The listing builds one solid part. Answer for the finished solid, in the listing's coordinates (mm). A direction names the side the tool comes from. Round coordinates to 2 decimals unless told otherwise and drop trailing zeros. Write each loop counter-clockwise with the first axis right and the second up, starting at its lowest first coordinate (ties: lowest second). Pieces come first, ordered by that corner, then holes.
Item 1: This flat-tipped pin is pushed along its axis until it touches: pin 1 (3 mm diameter, centred on x = 44.5, z = 173.5, fed in from -Y). Where does it stop, or does it pass through?
Item 2: For a pull along X with two mould halves and no side action, classify faces 1 (the face through (68, 0, 132)), 2 (the face through (59, 3, 267)) as +X half, -X half, draft (parallel to the pull), parting line (faces both ways), or undercut.
Item 3: A tool of negligible diameter and unlimited length cuts with its end or side. For faces 3 (the face through (59, 3, 0)), 4 (the face through (95.24, -13, 135)), from which of +Z, -Z, +X, -X, +Y, -Y can it reach the whole face along a straight path? Write none if from no direction.
Item 4: Find the intervals of material crossed by probe 1 along Y at (x, z) = (39, 163), in increasing order.
Item 5: Find section A-A on y = -11.5. Give the number of separate pieces and of enclosed holes in the cut face, then the cut area to 3 significant figures.
Item 6: Find section B-B on x = 53. Give the vertices of the cut face in (y, z).
Autodesk Inventor part; units mm, degrees
ref_plane "YZ Plane" through (0, 0, 0) normal (1, 0, 0) x (0, 1, 0)
ref_plane "XZ Plane" through (0, 0, 0) normal (0, 1, 0) x (-1, 0, 0)
ref_plane "XY Plane" through (0, 0, 0) normal (0, 0, 1) x (1, 0, 0)
sketch "Sketch4" plane through (0, 0, 0) normal (0, 0, 1) x (1, 0, 0)
  line L0 (0, 0) -> (97.04, 0)
  line L1 (97.04, 0) -> (97.04, 7.8)
  line L2 (97.04, 7.8) -> (0, 7.8)
  line L3 (0, 7.8) -> (0, 0)
  dimension "d15" = 97.04
  dimension "d16" = 7.8
extrude "Extrusion3" add sketch "Sketch4" along normal blind 267
sketch "Sketch5" plane through (0, 0, 267) normal (0, 0, 1) x (1, 0, 0)
  line L0 (0, 0) -> (97.04, 0)
  line L1 (0, 0) -> (1.8, 0)
  line L2 (1.8, 0) -> (1.8, -25.2)
  line L3 (1.8, -25.2) -> (0, -25.2)
  line L4 (0, -25.2) -> (0, 0)
  line L5 (9.7367, 0) -> (9.7367, -25.2)
  line L6 (7.9367, 0) -> (9.7367, 0)
  line L7 (7.9367, -25.2) -> (7.9367, 0)
  line L8 (9.7367, -25.2) -> (7.9367, -25.2)
  line L9 (17.6733, 0) -> (17.6733, -25.2)
  line L10 (15.8733, 0) -> (17.6733, 0)
  line L11 (15.8733, -25.2) -> (15.8733, 0)
  line L12 (17.6733, -25.2) -> (15.8733, -25.2)
  line L13 (25.61, 0) -> (25.61, -25.2)
  line L14 (23.81, 0) -> (25.61, 0)
  line L15 (23.81, -25.2) -> (23.81, 0)
  line L16 (25.61, -25.2) -> (23.81, -25.2)
  line L17 (33.5467, 0) -> (33.5467, -25.2)
  line L18 (31.7467, 0) -> (33.5467, 0)
  line L19 (31.7467, -25.2) -> (31.7467, 0)
  line L20 (33.5467, -25.2) -> (31.7467, -25.2)
  line L21 (41.4833, 0) -> (41.4833, -25.2)
  line L22 (39.6833, 0) -> (41.4833, 0)
  line L23 (39.6833, -25.2) -> (39.6833, 0)
  line L24 (41.4833, -25.2) -> (39.6833, -25.2)
  line L25 (49.42, 0) -> (49.42, -25.2)
  line L26 (47.62, 0) -> (49.42, 0)
  line L27 (47.62, -25.2) -> (47.62, 0)
  line L28 (49.42, -25.2) -> (47.62, -25.2)
  line L29 (57.3567, 0) -> (57.3567, -25.2)
  line L30 (55.5567, 0) -> (57.3567, 0)
  line L31 (55.5567, -25.2) -> (55.5567, 0)
  line L32 (57.3567, -25.2) -> (55.5567, -25.2)
  line L33 (65.2933, 0) -> (65.2933, -25.2)
  line L34 (63.4933, 0) -> (65.2933, 0)
  line L35 (63.4933, -25.2) -> (63.4933, 0)
  line L36 (65.2933, -25.2) -> (63.4933, -25.2)
  line L37 (73.23, 0) -> (73.23, -25.2)
  line L38 (71.43, 0) -> (73.23, 0)
  line L39 (71.43, -25.2) -> (71.43, 0)
  line L40 (73.23, -25.2) -> (71.43, -25.2)
  line L41 (81.1667, 0) -> (81.1667, -25.2)
  line L42 (79.3667, 0) -> (81.1667, 0)
  line L43 (79.3667, -25.2) -> (79.3667, 0)
  line L44 (81.1667, -25.2) -> (79.3667, -25.2)
  line L45 (89.1033, 0) -> (89.1033, -25.2)
  line L46 (87.3033, 0) -> (89.1033, 0)
  line L47 (87.3033, -25.2) -> (87.3033, 0)
  line L48 (89.1033, -25.2) -> (87.3033, -25.2)
  line L49 (97.04, 0) -> (97.04, -25.2)
  line L50 (95.24, 0) -> (97.04, 0)
  line L51 (95.24, -25.2) -> (95.24, 0)
  line L52 (97.04, -25.2) -> (95.24, -25.2)
  dimension "d19" = 1.8
  dimension "d20" = 25.2
  dimension "d23" = 7.9367
extrude "Extrusion4" add sketch "Sketch5" against normal up to surface (267 mm away)
properties part number "heat sink"
Check values:
1. pin 1: stops at y = 0
2. face 1: undercut
2. face 2: draft
3. face 3: -Z, +X, -X, +Y, -Y
3. face 4: +Z, -Z, -Y
4. probe 1: y = 0 to 7.8
5. separate pieces: 13
5. enclosed holes: 0
5. area: 6,250 mm2
6. outline: (0, 0) - (7.8, 0) - (7.8, 267) - (0, 267) - close
